Input: part model. Units: mm. Frame: model coordinates. Face numbers are marked on the shaded views. A direction names the side the tool comes from. Coordinates: 2 decimals unless noted, no trailing zeros. Loops run counter-clockwise (first coordinate to the right, second up) from the corner with the lowest first, then second, coordinate; pieces in that order, holes last. Notation, with made-up numbers: (-25, -13.75) - (33, -13.75) arc R17 cw to (33, 19.25) - close; hole circle Ø2 at (0.5, 62). An arc over 180 degrees is marked (long way). Use a Markdown table: item, result. Add a question column.
1. Access query for the marked faces 4, 5, 6 and 7. Directions: +Z, -Z, +X, -X, +Y, -Y. A direction counts if a zero-diameter tool reaches every point of the face in a straight line with its end or side. Return the directions, or none.
2. Contact query for flat-ended pins moving along their axis: P1, Ø2.5, axis at y = 12.5, z = 3.5, coming from the -X side; P2, Ø2, axis at x = 0.5, z = 2.5, coming from the +Y side; P3, Ø1.5, axis at x = -4, z = 2, coming from the -Y side. Output: stop coordinate, or through.
3. Section query C-C on z = 1.05. Return the cut outline in (x, y).
4. Section query B-B on y = 2. Return the cut outline in (x, z), then the cut area to 3 significant figures.
5. Draft query along Y for the marked faces 1, 2 and 3. Return one class per face: released by +Y, released by -Y, zero draft, split by the parting line, or undercut.
6. Ray query, L1, parallel to X at y = 3.5, z = 3.75; L2, parallel to X at y = 14, z = 3.75; L3, parallel to Y at x = -14, z = 3.35. Return the intervals inside material, ascending. Write a range as [from, to].
7. Section query A-A on x = 4. Return the cut outline in (y, z), then the cut area to 3 significant figures.
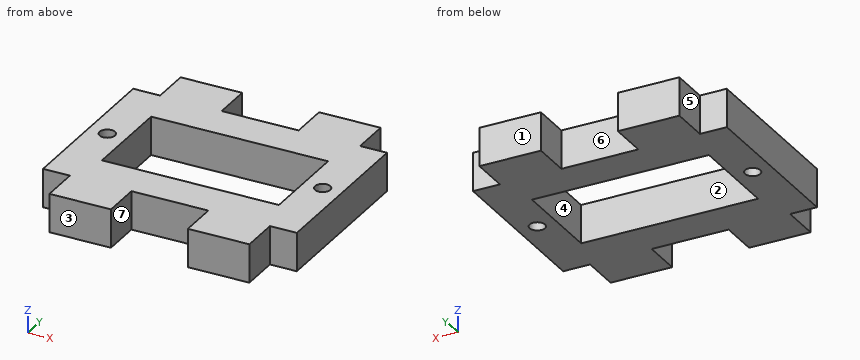
```python
from build123d import *

# Parameters (mm, degrees)
ESQUISSE1_R        = 1
ESQUISSE1_W        = 23
ESQUISSE1_H        = 12.000000104
BOSS_EXTRU_1_DEPTH = 5


with BuildPart() as part:
    # Esquisse1 → Boss.-Extru.1 (new body)
    with BuildSketch(Plane.XY):
        Polygon((5, 11), (5, 16), (13, 16), (13, 11), (16.5, 11), (16.5, -11), (13, -11), (13, -16), (5, -16), (5, -11), (-5, -11), (-5, -16), (-13, -16), (-13, -11), (-16.5, -11), (-16.5, 11), (-13, 11), (-13, 16), (-5, 16), (-5, 11), align=None)
        with Locations((-14, 0)):
            Circle(ESQUISSE1_R, mode=Mode.SUBTRACT)
        with Locations((14, 0)):
            Circle(ESQUISSE1_R, mode=Mode.SUBTRACT)
        Rectangle(ESQUISSE1_W, ESQUISSE1_H, mode=Mode.SUBTRACT)
    extrude(amount=BOSS_EXTRU_1_DEPTH)


solid = part.part
```
Resolved:
| question | item | result |
|---|---|---|
| 1 | face 4 | +Z, -Z |
| 1 | face 5 | +Z, -Z, -X, +Y |
| 1 | face 6 | +Z, -Z, +Y |
| 1 | face 7 | +Z, -Z, -Y |
| 2 | P1 | x = -13 |
| 2 | P2 | y = 11 |
| 2 | P3 | y = -11 |
| 3 | outline | (-16.5, -11) - (-13, -11) - (-13, -16) - (-5, -16) - (-5, -11) - (5, -11) - (5, -16) - (13, -16) - (13, -11) - (16.5, -11) - (16.5, 11) - (13, 11) - (13, 16) - (5, 16) - (5, 11) - (-5, 11) - (-5, 16) - (-13, 16) - (-13, 11) - (-16.5, 11) - close; hole circle Ø2 at (-14, 0); hole (-11.5, -6) - (11.5, -6) - (11.5, 6) - (-11.5, 6) - close; hole circle Ø2 at (14, 0) |
| 4 | outline | (-16.5, 0) - (-11.5, 0) - (-11.5, 5) - (-16.5, 5) - close; (11.5, 0) - (16.5, 0) - (16.5, 5) - (11.5, 5) - close |
| 4 | area | 50.0 mm² |
| 5 | face 1 | released by +Y |
| 5 | face 2 | undercut |
| 5 | face 3 | released by -Y |
| 6 | L1 | [-16.5, -11.5], [11.5, 16.5] |
| 6 | L2 | [-13, -5], [5, 13] |
| 6 | L3 | [-11, -1], [1, 11] |
| 7 | outline | (-11, 0) - (-6, 0) - (-6, 5) - (-11, 5) - close; (6, 0) - (11, 0) - (11, 5) - (6, 5) - close |
| 7 | area | 50.0 mm² |
